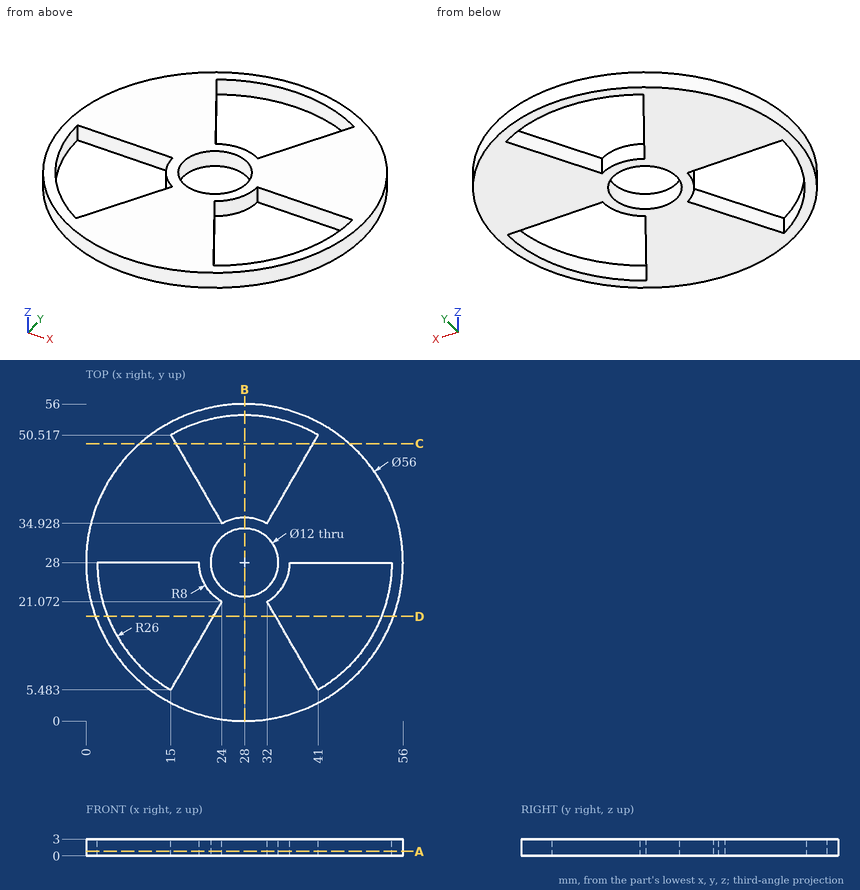
Input: dimensioned drawing with shaded views. Units: mm. Origin: part minimum x, y, z. Round coordinates to 2 decimals unless told otherwise and drop trailing zeros. Loops run counter-clockwise (first coordinate to the right, second up) from the corner with the lowest first, then second, coordinate; pieces in that order, holes last. Notation, with made-up numbers: (-24.75, 84.5) -> (-16.75, 84.5) arc R12 ccw to (-16.75, 106.5) -> close; hole circle Ø10 at (-13, -17). An arc over 180 degrees is marked (long way). Answer as a JSON object with one key per item and string values. Group by question number.
Q1. Section query C-C (y = 49). Output: boundary loops of the cut face in (x, z) (1 decimal).
Q2. Ray query, line 1 (Y direction, x = 28, z = 2.35); line 2 (X direction, y = 20, z = 2.45); line 3 (X direction, y = 24.5, z = 1.3) (1 decimal). Return the intervals inside material, ascending. Write a range as from..to.
Q3. Section query D-D (y = 18.5). Output: boundary loops of the cut face in (x, z) (1 decimal).
Q4. Section query B-B (x = 28). Output: boundary loops of the cut face in (y, z).
Q5. Contact query for flat-ended pins moving along their axis: P1, Ø0.9, axis at x = 40.5, z = 1, coming from the -Y side (1 decimal); P2, Ø1.5, axis at x = 41, z = 1, coming from the +Y side; P3, Ø1, axis at y = 21.5, z = 2, coming from the -X side. Output: stop coordinate, or through.
Q6. Section query A-A (z = 0.8). Output: boundary loops of the cut face in (x, y).
Completed:
{
 "1": {"outline": "(9.5, 0) -> (15.9, 0) -> (15.9, 3) -> (9.5, 3) -> close; (40.1, 0) -> (46.5, 0) -> (46.5, 3) -> (40.1, 3) -> close"},
 "2": {"line 1": "0..22, 34..36, 54..56", "line 2": "1.17..3.26, 23.38..32.62, 52.74..54.83", "line 3": "0.2..2.2, 20.8..23.1, 32.9..35.2, 53.8..55.8"},
 "3": {"outline": "(1.7, 0) -> (3.8, 0) -> (3.8, 3) -> (1.7, 3) -> close; (22.5, 0) -> (33.5, 0) -> (33.5, 3) -> (22.5, 3) -> close; (52.2, 0) -> (54.3, 0) -> (54.3, 3) -> (52.2, 3) -> close"},
 "4": {"outline": "(0, 0) -> (22, 0) -> (22, 3) -> (0, 3) -> close; (34, 0) -> (36, 0) -> (36, 3) -> (34, 3) -> close; (54, 0) -> (56, 0) -> (56, 3) -> (54, 3) -> close"},
 "5": {"P1": "y = 2.7", "P2": "y = 53.18", "P3": "x = 0.65"},
 "6": {"outline": "circle Ø56 at (28, 28); hole (2, 28) arc R26 ccw to (15, 5.48) -> (24, 21.07) arc R8 cw to (20, 28) -> close; hole (15, 50.52) -> (24, 34.93) arc R8 cw to (32, 34.93) -> (41, 50.52) arc R26 ccw to start; hole circle Ø12 at (28, 28); hole (32, 21.07) -> (41, 5.48) arc R26 ccw to (54, 28) -> (36, 28) arc R8 cw to start"}
}
